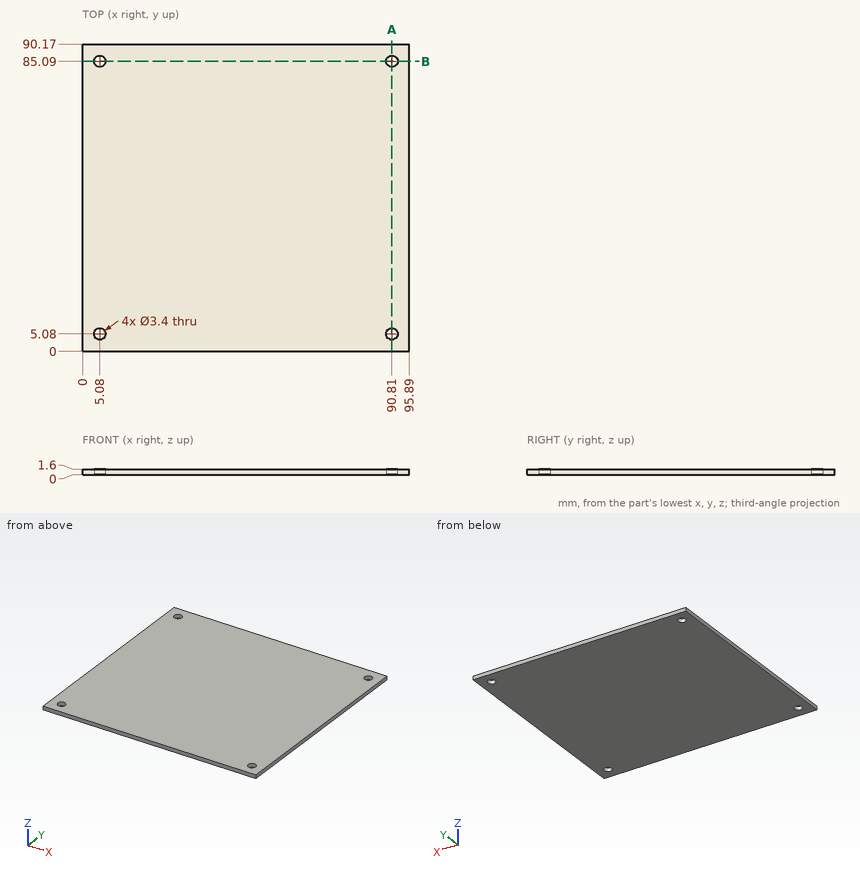
The drawing under review shows one solid part. Ordinate dimensions are in mm from its lowest x, y, z. Give positions to 0.01 mm unless a question says otherwise; leave off trailing zeros. Order: outer loops, then holes, each group sorted by start corner. A loop starts at its lowest first (then second) coordinate and runs counter-clockwise, first axis right, second up. Notation, with made-up numbers: M -37,76.25 L -25,76.25 A33 cw -25,114.25 Z; hole C 12,-37.5 d7. An arc over 180 degrees is marked long. One line per question, with ' | ' between items. Start each with the question number.
Q1. We need section A-A (x = 90.81). Write out the cut boundary in (y, z).
Q2. For L1, parallel to Y at x = 5.08, z = 0.6; L2, parallel to X at y = 5.08, z = 1.3; L3, parallel to X at y = 6.5, z = 1.3, list the stretches that pass through material, from the lowest coordinate up. Write a range as [from, to].
Q3. We need section B-B (y = 85.09). Write out the cut boundary in (x, z), plus the area to 3 significant figures.
Returned:
1) outline: M 0,0 L 3.38,0 L 3.38,1.6 L 0,1.6 Z; M 6.78,0 L 83.39,0 L 83.39,1.6 L 6.78,1.6 Z; M 86.79,0 L 90.17,0 L 90.17,1.6 L 86.79,1.6 Z
2) L1: [0, 3.38], [6.78, 83.39], [86.79, 90.17] | L2: [0, 3.38], [6.78, 89.11], [92.51, 95.89] | L3: [0, 4.15], [6.01, 89.88], [91.74, 95.89]
3) outline: M 0,0 L 3.38,0 L 3.38,1.6 L 0,1.6 Z; M 6.78,0 L 89.11,0 L 89.11,1.6 L 6.78,1.6 Z; M 92.51,0 L 95.89,0 L 95.89,1.6 L 92.51,1.6 Z | area: 143 mm2
